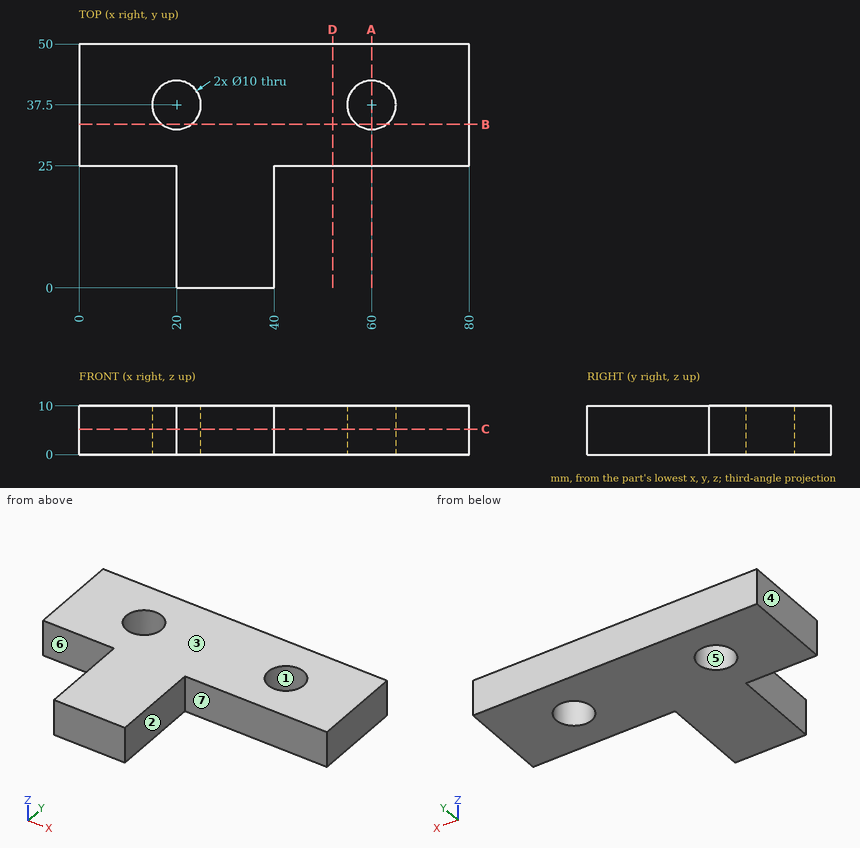
Geometry check sheet. Reference: drawing and pictorial views, mm from the part's lowest x, y, z. A direction names the side the tool comes from. Coordinates: 2 decimals unless noted, no trailing zeros. Order: outer loops, then holes, each group sorted by start corner. A loop starts at its lowest first (then second) coordinate and runs counter-clockwise, first axis right, second up.
1. Sectioned sample at A-A, the plane x = 60. Record the cut outline in (y, z).
Results found:
outline: (25, 0) - (32.5, 0) - (32.5, 10) - (25, 10) - close; (42.5, 0) - (50, 0) - (50, 10) - (42.5, 10) - close
2. Sectioned sample at C-C, the plane z = 5.25. Record the cut outline in (x, y).
Results found:
outline: (0, 25) - (20, 25) - (20, 0) - (40, 0) - (40, 25) - (80, 25) - (80, 50) - (0, 50) - close; hole circle Ø10 at (20, 37.5); hole circle Ø10 at (60, 37.5)
3. Sectioned sample at B-B, the plane y = 33.5. Record the cut outline in (x, z), and give its area (3 significant figures).
Results found:
outline: (0, 0) - (17, 0) - (17, 10) - (0, 10) - close; (23, 0) - (57, 0) - (57, 10) - (23, 10) - close; (63, 0) - (80, 0) - (80, 10) - (63, 10) - close
area: 680 mm2
4. Release check for a two-part mould opening along X. For the marked faces 1, 2, 3 and 4 record: +X half, -X half, draft (parallel to the pull), parting line (faces both ways), or undercut.
Results found:
face 1: undercut
face 2: +X half
face 3: draft
face 4: -X half
5. Set-up check for the marked faces 5, 6 and 7: record each of +Z, -Z, +X, -X, +Y, -Y from which the full face is reachable in a straight line by a thin tool's end or side.
Results found:
face 5: +Z, -Z
face 6: +Z, -Z, -X, -Y
face 7: +Z, -Z, +X, -Y
6. Go/stop test with flat-tipped pins: pin 1 Ø9 at (x, y) = (60, 37.5) entering from -Z; pin 2 Ø5 at (y, z) = (12, 3.5) entering from +X; pin 3 Ø5 at (x, z) = (13.5, 3.5) entering from -Y; pin 4 Ø1.5 at (y, z) = (13.5, 2) entering from -X. Record where each tip stops, or that it passes through.
Results found:
pin 1: passes through
pin 2: stops at x = 40
pin 3: stops at y = 25
pin 4: stops at x = 20
7. Scan lines: line 1 (X direction, y = 33.5, z = 0.5); line 2 (X direction, y = 35, z = 4); line 3 (Y direction, x = 60, z = 3.25). Record each from-to range of solid material in increasing order.
Results found:
line 1: x = 0 to 17, 23 to 57, 63 to 80
line 2: x = 0 to 15.67, 24.33 to 55.67, 64.33 to 80
line 3: y = 25 to 32.5, 42.5 to 50
8. Sectioned sample at D-D, the plane x = 52. Record the cut outline in (y, z).
Results found:
outline: (25, 0) - (50, 0) - (50, 10) - (25, 10) - close
